```python
from build123d import *
from build123d.topology import SkipClean

# Parameters (mm, degrees)
SKETCH_1_R          = 5
EXTRUDE_1_DEPTH     = 4
CUT_EXTRUDE_1_DEPTH = 10
SKETCH_3_R          = 1.2
CUT_EXTRUDE_2_DEPTH = 5


with BuildPart() as part:
    # 草图1 → 凸台-拉伸1 (new body)
    with BuildSketch(Plane.XY):
        with BuildLine():
            Line((10, 28.284271247), (10, 36))
            Line((10, 36), (-10, 36))
            Line((-10, 36), (-10, 28.284271247))
            ThreePointArc((-10, 28.284271247), (-25.980762114, 15), (-29.494897428, -5.481881586))
            Line((-29.494897428, -5.481881586), (-36.176914536, -9.339745962))
            Line((-36.176914536, -9.339745962), (-26.176914536, -26.660254038))
            Line((-26.176914536, -26.660254038), (-19.494897428, -22.802389662))
            ThreePointArc((-19.494897428, -22.802389662), (0, -30), (19.494897428, -22.802389662))
            Line((19.494897428, -22.802389662), (26.176914536, -26.660254038))
            Line((26.176914536, -26.660254038), (36.176914536, -9.339745962))
            Line((36.176914536, -9.339745962), (29.494897428, -5.481881586))
            ThreePointArc((29.494897428, -5.481881586), (25.980762114, 15), (10, 28.284271247))
        make_face()
        Circle(SKETCH_1_R, mode=Mode.SUBTRACT)
    extrude(amount=EXTRUDE_1_DEPTH)

    # 草图2 → 切除-拉伸1 (cut)
    with SkipClean():  # the faces are left unmerged after this step: merging them gives an invalid solid
        with BuildSketch(Plane(origin=(0, 0, 0), x_dir=(-1, 0, 0), z_dir=(0, 0, -1))):
            with BuildLine():
                Line((-7.5, 29.047375097), (-7.5, 36))
                Line((-7.5, 36), (-10, 36))
                Line((-10, 36), (-10, 28.284271247))
                ThreePointArc((-10, 28.284271247), (-8.758315013, 28.693063938), (-7.5, 29.047375097))
            make_face()
            with BuildLine():
                Line((7.5, 36), (7.5, 29.047375097))
                ThreePointArc((7.5, 29.047375097), (8.758315013, 28.693063938), (10, 28.284271247))
                Line((10, 28.284271247), (10, 36))
                Line((10, 36), (7.5, 36))
            make_face()
            with BuildLine():
                Line((-34.926914536, -11.504809472), (-28.905764747, -8.02849702))
                ThreePointArc((-28.905764747, -8.02849702), (-29.228079789, -6.761608673), (-29.494897428, -5.481881586))
                Line((-29.494897428, -5.481881586), (-36.176914536, -9.339745962))
                Line((-36.176914536, -9.339745962), (-34.926914536, -11.504809472))
            make_face()
            with BuildLine():
                Line((-26.176914536, -26.660254038), (-27.426914536, -24.495190528))
                Line((-27.426914536, -24.495190528), (-21.405764747, -21.018878077))
                ThreePointArc((-21.405764747, -21.018878077), (-20.469764776, -21.931455265), (-19.494897428, -22.802389662))
                Line((-19.494897428, -22.802389662), (-26.176914536, -26.660254038))
            make_face()
            with BuildLine():
                Line((36.176914536, -9.339745962), (34.926914536, -11.504809472))
                Line((34.926914536, -11.504809472), (28.905764747, -8.02849702))
                ThreePointArc((28.905764747, -8.02849702), (29.228079789, -6.761608673), (29.494897428, -5.481881586))
                Line((29.494897428, -5.481881586), (36.176914536, -9.339745962))
            make_face()
            with BuildLine():
                Line((27.426914536, -24.495190528), (21.405764747, -21.018878077))
                ThreePointArc((21.405764747, -21.018878077), (20.469764776, -21.931455265), (19.494897428, -22.802389662))
                Line((19.494897428, -22.802389662), (26.176914536, -26.660254038))
                Line((26.176914536, -26.660254038), (27.426914536, -24.495190528))
            make_face()
        extrude(amount=-CUT_EXTRUDE_1_DEPTH, mode=Mode.SUBTRACT)

    # 草图3 → 切除-拉伸2 (cut, symmetric)
    with SkipClean():  # the faces are left unmerged after this step: merging them gives an invalid solid
        with BuildSketch(Plane(origin=(0, 0, 0), x_dir=(-1, 0, 0), z_dir=(0, 0, -1))):
            with Locations(Location((0, 15, 0), (0, 0, 180))):
                Circle(SKETCH_3_R)
            with Locations(Location((12.990381057, -7.5, 0), (0, 0, 180))):
                Circle(SKETCH_3_R)
            with Locations(Location((-12.990381057, -7.5, 0), (0, 0, 180))):
                Circle(SKETCH_3_R)
        extrude(amount=CUT_EXTRUDE_2_DEPTH, both=True, mode=Mode.SUBTRACT)


solid = part.part
```
Read the model definition and answer for the solid it produces. Units are mm, in the model's axes. A direction names the side the tool comes from. Give positions to 0.01 mm unless a question says otherwise; leave off trailing zeros. Order: outer loops, then holes, each group sorted by start corner. A loop starts at its lowest first (then second) coordinate and runs counter-clockwise, first axis right, second up. Notation, with made-up numbers: (45.25, 62.5) -> (81.25, 62.5) arc R22 ccw to (81.25, 90.5) -> close; hole circle Ø9 at (-34, 49.5). An arc over 180 degrees is marked (long way). Write item = value, one per line.
1. A cutting plane is placed at C-C, the plane z = 2.9. Write down the section's boundary in (x, y).
Numbers:
outline = (-34.93, -11.5) -> (-27.43, -24.5) -> (-21.41, -21.02) arc R30 ccw to (21.41, -21.02) -> (27.43, -24.5) -> (34.93, -11.5) -> (28.91, -8.03) arc R30 ccw to (7.5, 29.05) -> (7.5, 36) -> (-7.5, 36) -> (-7.5, 29.05) arc R30 ccw to (-28.91, -8.03) -> close; hole circle Ø2.4 at (-12.99, -7.5); hole circle Ø10 at (0, 0); hole circle Ø2.4 at (0, 15); hole circle Ø2.4 at (12.99, -7.5)
2. A cutting plane is placed at B-B, the plane x = 0. Write down the section's boundary in (y, z).
Numbers:
outline = (-30, 0) -> (-5, 0) -> (-5, 4) -> (-30, 4) -> close; (5, 0) -> (13.8, 0) -> (13.8, 4) -> (5, 4) -> close; (16.2, 0) -> (36, 0) -> (36, 4) -> (16.2, 4) -> close
3. For faces 5 (the face through (31.96, -9.79, 1.97)), 6 (the face through (7.5, 32, 2)), 7 (the face through (24.46, -22.78, 1.97)), 8 (the face through (-7.5, 33, 2)), determine the directions among +Z, -Z, +X, -X, +Y, -Y from which every point of the face is accessible in a straight line to the end or side of a thin tool.
Numbers:
face_5 = +Z, -Z, +X
face_6 = +Z, -Z, +X, +Y
face_7 = +Z, -Z, -Y
face_8 = +Z, -Z, -X, +Y
4. The mould has two halves that part along Y. Classify faces 1 (the face through (-31.96, -9.79, 1.97)), 2 (the face through (0, 36, 2)), 3 (the face through (31.124, -18.091, 1.972)), 4 (the face through (7, 3, 0)): +Y half, -Y half, draft (parallel to the pull), parting line (faces both ways), or undercut.
Numbers:
face_1 = undercut
face_2 = +Y half
face_3 = -Y half
face_4 = draft
5. Given pin 1 (2 mm diameter, centred on x = -2.5, y = -3.5, fed in from -Z); pin 2 (1.5 mm diameter, centred on y = -12.5, z = 3.5, fed in from -X); pin 3 (1.2 mm diameter, centred on y = 34, z = 3, fed in from -X); pin 4 (2 mm diameter, centred on x = 17.5, z = 1.5, fed in from -Y), each flat-ended and moving along its own axis, determine where each tip first touches the part or whether it passes through.
Numbers:
pin_1 = 0
pin_2 = -34.79
pin_3 = -7.5
pin_4 = -25.05
6. A cutting plane is placed at A-A, the plane y = 0. Write down the section's boundary in (x, z).
Numbers:
outline = (-30, 0) -> (-5, 0) -> (-5, 4) -> (-30, 4) -> close; (5, 0) -> (30, 0) -> (30, 4) -> (5, 4) -> close
7. A cutting plane is placed at D-D, the plane y = -22. Write down the section's boundary in (x, z).
Numbers:
outline = (-28.87, 0) -> (-23.11, 0) -> (-23.11, 4) -> (-28.87, 4) -> close; (-20.4, 0) -> (20.4, 0) -> (20.4, 4) -> (-20.4, 4) -> close; (23.11, 0) -> (28.87, 0) -> (28.87, 4) -> (23.11, 4) -> close
8. Straight lines are drawn through the part: line 1 along Y through (x, z) = (0, 1); line 2 along X through (y, z) = (-7.5, 1.4); line 3 along Y through (x, z) = (21, 0.4). For each, find the intervals that lie inside material, in ascending order.
Numbers:
line_1 = -30 to -5, 5 to 13.8, 16.2 to 36
line_2 = -29.05 to -14.19, -11.79 to 11.79, 14.19 to 29.05
line_3 = -21.42 to 21.42
